Model file for the job. Use its own axes, mm. A direction names the side the tool comes from. Coordinates: 2 decimals unless noted, no trailing zeros. Loops run counter-clockwise (first coordinate to the right, second up) from the corner with the lowest first, then second, coordinate; pieces in that order, holes last. Notation, with made-up numbers: M 28.25,33.5 L 36.25,33.5 A23 cw 36.25,60.5 Z; hole C -10,13.5 d6. An arc over 180 degrees is marked long. Write item = value, one per line. Start each with the question number.
from build123d import *

# Parameters (mm, degrees)
F1_DEPTH = 55
F3_DEPTH = 60
F5_D     = 4.2
F7_D     = 5
F8_SIZE2 = 2
F8_SIZE  = 2


with BuildPart() as f1:
    # F0 (on Right) → F1 (new body)
    with BuildSketch(Plane.YZ):
        Polygon((-12.5, 0), (0, 0), (0, 15), (-22, 15), (-22, 10), (-12.5, 10), align=None)
    extrude(amount=F1_DEPTH)

    # F2 (on face) → F3 (cut)
    with BuildSketch(Plane.XY.offset(15)):
        with BuildLine():
            Line((34.9833147735, 0), (20.0166852265, 0))
            ThreePointArc((20.0166852265, 0), (27.5, -7), (34.9833147735, 0))
        make_face()
        with BuildLine():
            ThreePointArc((34.9833147735, 0), (34.9958275328, 0.2498608403), (35, 0.5))
            ThreePointArc((35, 0.5), (27.2498608403, 7.9958275328), (20.0166852265, 0))
            Line((20.0166852265, 0), (34.9833147735, 0))
        make_face()
    extrude(amount=-F3_DEPTH, mode=Mode.SUBTRACT)

    # F5 (through all)
    with Locations(Plane.XY.offset(15)):
        with Locations((25, -18), (45, -18)):
            Hole(F5_D / 2)

    # F7 (through all)
    with Locations(Plane(origin=(0, 0, 0), x_dir=(-1, 0, 0), z_dir=(0, 1, 0))):
        with Locations((-10.413300395, 7.5), (-45.413300395, 7.5)):
            Hole(F7_D / 2)

    # F8
    f8_edges = [f1.edges().sort_by_distance(p)[0] for p in [
        (0, -22, 12.5),
        (55, -22, 12.5),
    ]]
    chamfer(f8_edges, length=F8_SIZE, length2=F8_SIZE2)


solid = f1.part
Item 1: Cut at B-B (z = 7.5). Give the cut face in (x, y), plus the area to 3 significant figures.
Item 2: Cut at D-D (x = 25). Give the cut face in (y, z), plus the area to 3 significant figures.
Item 3: Probe L1, parallel to X at y = -8.75, z = 7.5; L2, parallel to X at y = -19.75, z = 10.5; L3, parallel to Y at x = 45, z = 11.4. List the from-to ranges inside material, lowest first.
Item 4: Cut at C-C (y = -9.75). Give the cut face in (x, z), plus the area to 3 significant figures.
Item 5: 3-axis set-ups, long thin cutter, end or side, ignore diameter. For faces 4 (the cylindrical face through (8.43, -6.34, 5.98)), 5 (the flat face through (27, -12.5, 5)): which of +Z, -Z, +X, -X, +Y, -Y reach the whole face in a straight line?
Item 6: Pull direction X, two halves, no side cores. Call faces 1 (the flat face through (54, -21, 13)), 2 (the cylindrical face through (25.273, -15.918, 12.465)), 3 (the flat face through (27, -8, 0)): +X half, -X half, draft (parallel to the pull), parting line (faces both ways), or undercut.
Item 7: Pin check, flat tips, straight feed: pin 1 Ø3 at (x, z) = (16.5, 6.5) entering from -Y; pin 2 Ø2.5 at (x, y) = (45, -18) entering from -Z. Stop position of each tip, or through.
Item 8: Cut at A-A (y = -18). Give the cut face in (x, z).
Reported:
q1.outline = M 0,-12.5 L 7.91,-12.5 L 7.91,0 L 0,0 Z; M 12.91,-12.5 L 42.91,-12.5 L 42.91,0 L 34.98,0 A7.5 cw 20.02,0 L 12.91,0 Z; M 47.91,-12.5 L 55,-12.5 L 55,0 L 47.91,0 Z
q1.area = 482 mm^2
q2.outline = M -22,10 L -20.1,10 L -20.1,15 L -22,15 Z; M -15.9,10 L -12.5,10 L -12.5,0 L -6.57,0 L -6.57,15 L -15.9,15 Z
q2.area = 115 mm^2
q3.L1 = 0 to 7.91, 12.91 to 42.91, 47.91 to 55
q3.L2 = 0 to 23.84, 26.16 to 43.84, 46.16 to 55
q3.L3 = -22 to -20.1, -15.9 to 0
q4.outline = M 0,0 L 55,0 L 55,15 L 0,15 Z; hole C 10.41,7.5 d5; hole C 45.41,7.5 d5
q4.area = 786 mm^2
q5.face_4 = +Y, -Y
q5.face_5 = -Z, +X, -X, -Y
q6.face_1 = +X half
q6.face_2 = undercut
q6.face_3 = draft
q7.pin_1 = -12.5
q7.pin_2 = through
q8.outline = M 0,10 L 22.9,10 L 22.9,15 L 0,15 Z; M 27.1,10 L 42.9,10 L 42.9,15 L 27.1,15 Z; M 47.1,10 L 55,10 L 55,15 L 47.1,15 Z
